For this review, take the finished solid that the model builds, in its own axes (mm). A direction names the side the tool comes from. Coordinates: 2 decimals unless noted, no trailing zeros. Write each loop counter-clockwise with the first axis right and the second up, starting at its lowest first coordinate (ties: lowest second). Pieces come first, ordered by that corner, then holes.
Autodesk Inventor part; units mm, degrees
ref_plane "YZ Plane" through (0, 0, 0) normal (1, 0, 0) x (0, 1, 0)
ref_plane "XZ Plane" through (0, 0, 0) normal (0, 1, 0) x (-1, 0, 0)
ref_plane "XY Plane" through (0, 0, 0) normal (0, 0, 1) x (1, 0, 0)
sketch "Sketch1" plane through (0, 0, 0) normal (0, 0, 1) x (1, 0, 0)
  circle A0 centre (-0.7749, 5.5) radius 1
  circle A1 centre (7.2251, 5.5) radius 1
  circle A2 centre (-0.7749, -5.5) radius 1
  circle A3 centre (7.2251, -5.5) radius 1
  line L0 (11.2251, -3) -> (-3.7749, -3)
  line L1 (-3.7749, -3) -> (-3.7749, 3)
  line L2 (-3.7749, 3) -> (11.2251, 3)
  line L3 (11.2251, 3) -> (11.2251, 8)
  line L4 (11.2251, 8) -> (-8.528, 8)
  arc A4 (-8.528, -8) -> (-8.528, 8) centre (-18.7749, 0) ccw
  line L5 (-8.528, -8) -> (11.2251, -8)
  line L6 (11.2251, -8) -> (11.2251, -3)
  point P0 (0, 0)
extrude "Extrusion1" add sketch "Sketch1" along normal blind 3
sketch "Sketch2" plane through (0, 0, 3) normal (0, 0, 1) x (1, 0, 0)
  line L0 (11.2251, -8) -> (11.2251, -3)
  line L1 (11.2251, -3) -> (-3.7749, -3)
  line L2 (-3.7749, -3) -> (-3.7749, 3)
  line L3 (-3.7749, 3) -> (11.2251, 3)
  line L4 (11.2251, 3) -> (11.2251, 8)
  line L5 (11.2251, 8) -> (-8.528, 8)
  arc A0 (-8.528, -8) -> (-8.528, 8) centre (-18.7749, 0) ccw
  line L6 (-8.528, -8) -> (11.2251, -8)
  circle A1 centre (-0.7749, 5.5) radius 1
  circle A2 centre (7.2251, 5.5) radius 1
  circle A3 centre (-0.7749, -5.5) radius 1
  circle A4 centre (7.2251, -5.5) radius 1
  line L7 (11.2251, -8) -> (11.2251, -3)
  line L8 (11.2251, 3) -> (11.2251, 8)
  line L9 (11.2251, -8) -> (11.2251, 8)
  point P0 (0, 0)
extrude "Extrusion2" add sketch "Sketch2" along normal blind 5
chamfer "Chamfer1" distance 3 angle 45 1 edges at (-5.7749, 0, 8)
fillet "Fillet1" radius 1 2 edges at (-6.817, -8, 6.3872) (-6.817, 8, 6.3872)
chamfer "Chamfer2" distance 2 angle 45 1 edges at (11.2251, 0, 8)
fillet "Fillet2" radius 2 2 edges at (10.2251, -8, 7) (10.2251, 8, 7)
thicken "Thicken1" operation add thickness 0.08 both sides no extend neighbours yes toward (0, 1, 0) faces at (1.2251, 3, 1)
thicken "Thicken2" operation add thickness 0.08 both sides no extend neighbours yes toward (0, -1, 0) faces at (6.2251, -3, 1)
properties part number "armtip_2_mod"
Q1. Add section C-C (y = -5.5). Give the number of separate pieces and of enclosed holes in the cut face, then the cut area to 3 significant figures.
Ans:
separate pieces: 3
enclosed holes: 0
area: 107 mm2
Q2. Add section B-B (x = -2.5). State the section outline as (y, z) points.
Ans:
outline: (-8, 0) - (-3.08, 0) - (-3.08, 3) - (3.08, 3) - (3.08, 0) - (8, 0) - (8, 8) - (-8, 8) - close
Q3. Tool access review of faces 1 (the flat face through (11.225, 0, 4)), 2 (the flat face through (4, 0, 3)): name each direction out of +Z, -Z, +X, -X, +Y, -Y from which nothing blocks a thin tool from reaching the whole face with its end or side.
Ans:
face 1: +Z, -Z, +X, +Y, -Y
face 2: -Z, +X
Q4. Add section A-A (z = 1.75). State the section outline as (x, y) points, then the cut area to 3 significant figures.
Ans:
outline: (-8.53, -8) - (11.23, -8) - (11.23, -3.08) - (-3.77, -3.08) - (-3.77, 3.08) - (11.23, 3.08) - (11.23, 8) - (-8.53, 8) arc R13 cw to start; hole circle Ø2 at (-0.77, -5.5); hole circle Ø2 at (-0.77, 5.5); hole circle Ø2 at (7.23, -5.5); hole circle Ø2 at (7.23, 5.5)
area: 181 mm2
Q5. For probe 1 along Y at (x, z) = (-0.75, 6.5); probe 2 along Y at (x, z) = (-3, 1.5); probe 3 along Y at (x, z) = (-1.5, 1), list the stretches that pass through material, from the lowest coordinate up.
Ans:
probe 1: y = -8 to -6.5, -4.5 to 4.5, 6.5 to 8
probe 2: y = -8 to -3.08, 3.08 to 8
probe 3: y = -8 to -6.19, -4.81 to -3.08, 3.08 to 4.81, 6.19 to 8
Q6. Draft analysis for pull direction X (two halves, no side actions). For faces 3 (the flat face through (4, 3.08, 1)), 4 (the cylindrical face through (7.09, 4.51, 3.94)), 5 (the cylindrical face through (9.643, 7.651, 6.35)), state which applies: +X half, -X half, draft (parallel to the pull), parting line (faces both ways), or undercut.
Ans:
face 3: draft
face 4: undercut
face 5: +X half
Q7. Clearance check with flat-ended pins moving along their axes: pin 1 Ø5 at (x, y) = (1.5, 6) entering from -Z; pin 2 Ø3.5 at (y, z) = (-1, 1) entering from +X; pin 3 Ø1 at (y, z) = (4.5, 1.5) entering from -X. State where each tip first meets the part, or that it passes through.
Ans:
pin 1: stops at z = 0
pin 2: stops at x = -3.77
pin 3: stops at x = -6.77
